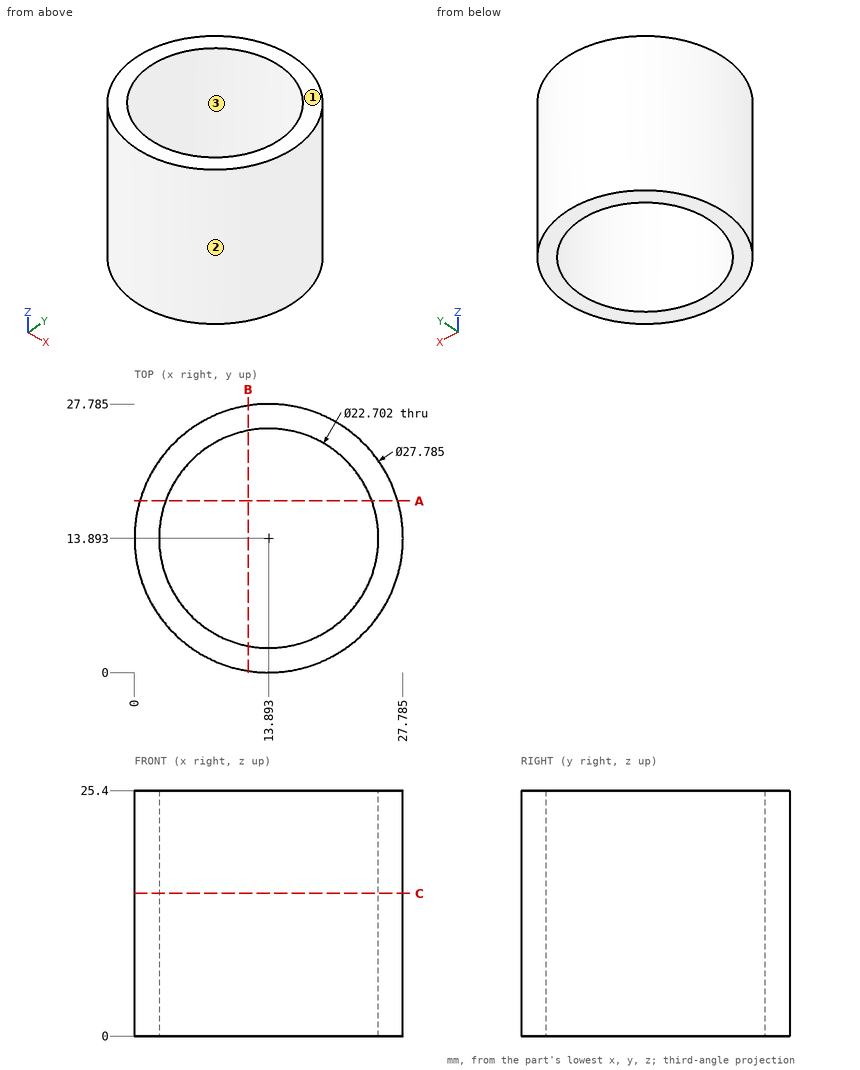
Here's the drawing with two shaded views (mm, measured from the low corner). I have some questions. Coordinates: 2 decimals unless noted, no trailing zeros. Loops run counter-clockwise (first coordinate to the right, second up) from the corner with the lowest first, then second, coordinate; pieces in that order, holes last. Notation, with made-up numbers: M -33,47 L 26,47 A22 cw 26,71 Z; hole C 27,13 d10. An arc over 180 degrees is marked long. Return JSON: item names as keys, results as strings. Group by question number.
Item 1: Imagine slicing it at B-B (x = 11.75). Please give me the cut outline in (y, z) (1 decimal), and give its area (3 significant figures).
Item 2: Imagine slicing it at C-C (z = 14.75). Please give me the cut outline in (x, y) (1 decimal).
Item 3: Imagine slicing it at A-A (y = 17.75). Please give me the cut outline in (x, z), and give its area (3 significant figures).
Item 4: Thinking about a two-plate mould opening in X: for the marked faces 1, 2 and 3, which applies, released by +X, released by -X, zero draft, split by the parting line, or undercut?
Item 5: If I drill on L1, parallel to X at y = 8, z = 5.5 (1 decimal); L2, parallel to Y at x = 12, z = 21.25 (1 decimal); L3, parallel to X at y = 6.5, z = 15 (1 decimal), over which ranges is the centre line in solid material (lowest first)? Write a range as from..to.
Item 6: I'm going to push flat-ended pins straight in: pin 1 Ø10 at (y, z) = (21.5, 2.5) entering from -X; pin 2 Ø2 at (y, z) = (19, 8.5) entering from +X; pin 3 Ø3 at (y, z) = (25, 18) entering from +X. Where does each tip first touch, or does it pass through?
Verdict:
{
 "1": {"outline": "M 0.2,0 L 2.7,0 L 2.7,25.4 L 0.2,25.4 Z; M 25,0 L 27.6,0 L 27.6,25.4 L 25,25.4 Z", "area": "131 mm^2"},
 "2": {"outline": "C 13.9,13.9 d27.8; hole C 13.9,13.9 d22.7"},
 "3": {"outline": "M 0.55,0 L 3.22,0 L 3.22,25.4 L 0.55,25.4 Z; M 24.57,0 L 27.24,0 L 27.24,25.4 L 24.57,25.4 Z", "area": "136 mm^2"},
 "4": {"face 1": "zero draft", "face 2": "split by the parting line", "face 3": "undercut"},
 "5": {"L1": "x = 1.3..4.2, 23.6..26.5", "L2": "y = 0.1..2.7, 25.1..27.7", "L3": "x = 2.1..5.3, 22.5..25.7"},
 "6": {"pin 1": "stops at x = 0.25", "pin 2": "stops at x = 27.16", "pin 3": "stops at x = 23.93"}
}
